```python
from build123d import *

# Parameters (mm, degrees)
FILLET1_R              = 8
M10_TAPPED_HOLE1_D     = 8.5
M10_TAPPED_HOLE1_DEPTH = 10
M10_TAPPED_HOLE1_TIP   = 2.553657631
M25X1_5_TAPPED_HOLE1_D = 23.5


with BuildPart() as part:
    # Sketch2 → Revolve1 (revolve)
    with BuildSketch(Plane.XY, mode=Mode.PRIVATE) as revolve1_sk:
        with BuildLine():
            Line((19.595917942, 0), (31, 0))
            Line((31, 0), (31, 20))
            Line((31, 20), (23, 46))
            Line((23, 46), (0, 46))
            Line((0, 46), (0, 4))
            ThreePointArc((0, 4), (10, 2.989794856), (19.595917942, 0))
        make_face()
    revolve(revolve1_sk.sketch.rotate(Axis((0, 46, 0), (0, -1, 0)), 90), axis=Axis((0, 46, 0), (0, -1, 0)))

    # Fillet1
    fillet1_edges = [part.edges().sort_by_distance(p)[0] for p in [
        (0, 46, -23),
    ]]
    fillet(fillet1_edges, radius=FILLET1_R)

    # M10 Tapped Hole1
    with Locations(Plane(origin=(-0.142010422, 30.849228359, 27.66141136), x_dir=(0, 0.955777919374, -0.294089389196), z_dir=(-0.00490679199, 0.294085848838, 0.955766413359))):
        with Locations((0, 0)):
            Hole(M10_TAPPED_HOLE1_D / 2, depth=M10_TAPPED_HOLE1_DEPTH)
            with Locations((0, 0, -(M10_TAPPED_HOLE1_DEPTH + M10_TAPPED_HOLE1_TIP / 2))):  # 118° drill point
                Cone(0, M10_TAPPED_HOLE1_D / 2, M10_TAPPED_HOLE1_TIP, mode=Mode.SUBTRACT)

    # M25x1.5 Tapped Hole1 (through all)
    with Locations(Plane.ZX.offset(46)):
        with Locations((0, 0)):
            Hole(M25X1_5_TAPPED_HOLE1_D / 2)


solid = part.part
```
Source: CAD feature listing. Evaluate the final solid. Frame: model axes, mm. Round coordinates to 2 decimals unless told otherwise and drop trailing zeros. Write each loop counter-clockwise with the first axis right and the second up, starting at its lowest first coordinate (ties: lowest second). Pieces come first, ordered by that corner, then holes. Notation, with made-up numbers: M 40.5,63 L 50.5,63 A25 cw 50.5,86 Z; hole C -3.5,-29 d11. An arc over 180 degrees is marked long. Answer as a JSON object with one key per item and string values. Group by question number.
(1) Mould query, pull axis X, two halves, no side actions, for faces 1 (the flat face through (20, 0, 0)), 2 (the cylindrical face through (3.529, 23.996, -11.207)), 3 (the conical face through (-7.73, 37.1, 24.55)), 4 (the conical face through (-0.58, 26.77, 16.24)). Classes: +X half, -X half, draft (parallel to the pull), parting line (faces both ways), or undercut.
(2) Section query C-C on y = 37.5. Output: boundary loops of the cut face in (x, z), then the cut area to 3 significant figures.
(3) Ray query, line 1 (X direction, y = 13.5, z = 0); line 2 (Z direction, x = -0.5, y = 19.5); line 3 (Z direction, x = -2.5, y = 24). Return the intervals inside material, ascending. Write a range as [from, to].
(4) Section query A-A on z = 0. Output: boundary loops of the cut face in (x, y), then the cut area to 3 significant figures.
(5) First-contact query: pin 1 (4 mm diameter, centred on x = 5, y = 32, fed in from +Z); pin 2 (1.5 mm diameter, centred on y = 31.5, z = -10, fed in from +X); pin 3 (2 mm diameter, centred on x = 6, y = 5, fed in from -Z). Flat tips, straight axial feed; report the tip coordinate or a pass-through.
(6) Section query B-B on y = 4. Output: boundary loops of the cut face in (x, z).
Computed values:
{
 "1": {"face 1": "draft", "face 2": "undercut", "face 3": "parting line", "face 4": "undercut"},
 "2": {"outline": "C 0,0 d51.23; hole C 0,0 d23.5", "area": "1,630 mm^2"},
 "3": {"line 1": "[-31, -11.75], [11.75, 31]", "line 2": "[-31, -11.74], [11.74, 31]", "line 3": "[-29.66, -11.48], [11.48, 29.66]"},
 "4": {"outline": "M -31,0 L -19.6,0 A50 cw -11.75,2.6 L -11.75,46 L -17.09,46 A8 ccw -24.74,40.35 L -31,20 Z; M 11.75,2.6 A50 cw 19.6,0 L 31,0 L 31,20 L 24.74,40.35 A8 ccw 17.09,46 L 11.75,46 Z", "area": "1,530 mm^2"},
 "5": {"pin 1": "z = 27.55", "pin 2": "x = 25.95", "pin 3": "z = -30.59"},
 "6": {"outline": "C 0,0 d62; hole C 0,0 d23.5"}
}
